from build123d import *

# Parameters (mm, degrees)
SKETCH1_W                = 3
SKETCH1_H                = 10
BOSS_EXTRUDE1_DEPTH      = 4
SKETCH2_W                = 3
SKETCH2_H                = 10
BOSS_EXTRUDE2_DEPTH      = 10
FILLET1_R                = 5
M3_CLEARANCE_HOLE1_D     = 3.4
M3_CLEARANCE_HOLE1_DEPTH = 70
M3_CLEARANCE_HOLE1_TIP   = 1.021463052
SKETCH6_W                = 10
SKETCH6_H                = 4
BOSS_EXTRUDE3_DEPTH      = 2
M3_CLEARANCE_HOLE2_D     = 3.4
M3_CLEARANCE_HOLE2_DEPTH = 70
M3_CLEARANCE_HOLE2_TIP   = 1.021463052
M3_CLEARANCE_HOLE3_D     = 3.4
M3_CLEARANCE_HOLE3_DEPTH = 70
M3_CLEARANCE_HOLE3_TIP   = 1.021463052


with BuildPart() as part:
    # Sketch1 → Boss-Extrude1 (new body)
    with BuildSketch(Plane.XY):
        Polygon((0, 15), (0, 0), (3.241791175, 0), (3.241791175, 10), (6.241791175, 10), (6.241791175, 0), (10, 0), (10, 15), align=None)
        with Locations((4.741791175, 5)):
            Rectangle(SKETCH1_W, SKETCH1_H)
    extrude(amount=BOSS_EXTRUDE1_DEPTH)

    # Sketch2 → Boss-Extrude2 (add)
    with BuildSketch(Plane.XY.offset(4)):
        with Locations((5, 5)):
            Rectangle(SKETCH2_W, SKETCH2_H)
    extrude(amount=BOSS_EXTRUDE2_DEPTH)

    # Fillet1
    fillet1_edges = [part.edges().sort_by_distance(p)[0] for p in [
        (5, 0, 14),
        (5, 10, 14),
    ]]
    fillet(fillet1_edges, radius=FILLET1_R - 0.0001)  # a hair under: the kernel refuses the full size

    # M3 Clearance Hole1
    with Locations(Plane.XY.offset(4)):
        with Locations((5, 13.5), (12.547675822, 14.055863144)):
            Hole(M3_CLEARANCE_HOLE1_D / 2, depth=M3_CLEARANCE_HOLE1_DEPTH)
            with Locations((0, 0, -(M3_CLEARANCE_HOLE1_DEPTH + M3_CLEARANCE_HOLE1_TIP / 2))):  # 118° drill point
                Cone(0, M3_CLEARANCE_HOLE1_D / 2, M3_CLEARANCE_HOLE1_TIP, mode=Mode.SUBTRACT)

    # Sketch6 → Boss-Extrude3 (add)
    with BuildSketch(Plane(origin=(0, 15, 0), x_dir=(1, 0, 0), z_dir=(0, 1, 0))):
        with Locations((5, -2)):
            Rectangle(SKETCH6_W, SKETCH6_H)
    extrude(amount=BOSS_EXTRUDE3_DEPTH)

    # M3 Clearance Hole2
    with Locations(Plane.XY.offset(4)):
        with Locations((5, 13.5)):
            Hole(M3_CLEARANCE_HOLE2_D / 2, depth=M3_CLEARANCE_HOLE2_DEPTH)
            with Locations((0, 0, -(M3_CLEARANCE_HOLE2_DEPTH + M3_CLEARANCE_HOLE2_TIP / 2))):  # 118° drill point
                Cone(0, M3_CLEARANCE_HOLE2_D / 2, M3_CLEARANCE_HOLE2_TIP, mode=Mode.SUBTRACT)

    # M3 Clearance Hole3
    with Locations(Plane(origin=(6.5, 0, 0), x_dir=(0, 0, -1), z_dir=(1, 0, 0))):
        with Locations((-10, 5)):
            Hole(M3_CLEARANCE_HOLE3_D / 2, depth=M3_CLEARANCE_HOLE3_DEPTH)
            with Locations((0, 0, -(M3_CLEARANCE_HOLE3_DEPTH + M3_CLEARANCE_HOLE3_TIP / 2))):  # 118° drill point
                Cone(0, M3_CLEARANCE_HOLE3_D / 2, M3_CLEARANCE_HOLE3_TIP, mode=Mode.SUBTRACT)


solid = part.part
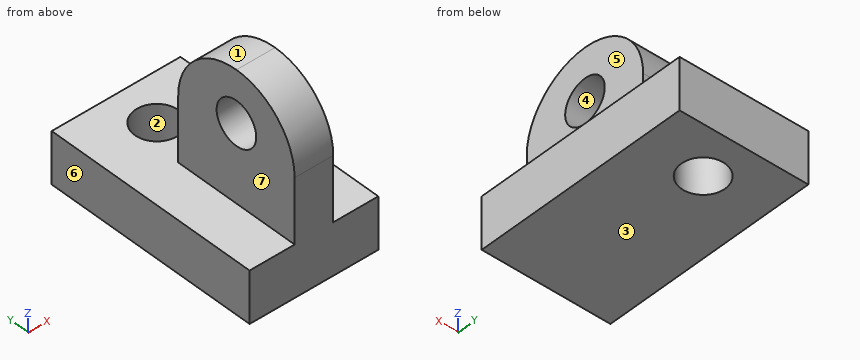
Here's how the part is built. I have some questions about the finished solid (model axes, mm). Face numbers are marked on the shaded views. A direction names the side the tool comes from. Round coordinates to 2 decimals unless told otherwise and drop trailing zeros. Write each loop counter-clockwise with the first axis right and the second up, starting at its lowest first coordinate (ties: lowest second). Pieces come first, ordered by that corner, then holes.
1. Will these pins go through, and if not, where does the flat tip stop? pin 1 Ø1.5 at (x, y) = (2, 14) entering from +Z; pin 2 Ø2.5 at (x, z) = (4.5, 6) entering from +Y; pin 3 Ø5.5 at (y, z) = (5, 10) entering from -X.
2. If we mould it in two halves opening along Z, with no side actions, what happens to the marked faces 1, 2, 3 and 4? For each: released by +Z, released by -Z, zero draft, split by the parting line, or undercut.
3. Suppose I cut it at A-A (x = 5). State how many separate pieces and enclosed holes the cut face has, and give its area (3 significant figures).
4. I need wall thicknesses on L1, parallel to Y at x = 5, z = 2.95; L2, parallel to Z at x = 7.75, y = 14.25; L3, parallel to Y at x = 6, z = 5.5. Which ranges of each line are inside material? Lowest first, please.
5. Suppose I cut it at C-C (z = 11.5). List the corners of the cut face in (x, y) for me.
6. Suppose I cut it at B-B (y = 13.5). List the corners of the cut face in (x, z) for me, and give its area (3 significant figures).
7. Suppose I cut it at D-D (z = 3.75). List the corners of the cut face in (x, y) for me, and give its area (3 significant figures).
8. For the marked faces 5, 6 and 7, which set-ups out of +Z, -Z, +X, -X, +Y, -Y let a thin tool reach every point of the face, with its end or its side?
Answer sheet:
1. pin 1: stops at z = 4
1. pin 2: stops at y = 10
1. pin 3: stops at x = 3.5
2. face 1: released by +Z
2. face 2: zero draft
2. face 3: released by -Z
2. face 4: undercut
3. separate pieces: 2
3. enclosed holes: 1
3. area: 135 mm2
4. L1: y = 0 to 11.8, 15.2 to 17
4. L2: z = 0 to 4
4. L3: y = 0 to 10
5. outline: (3.5, 0.67) - (6.5, 0.67) - (6.5, 4.2) - (3.5, 4.2) - close; (3.5, 5.8) - (6.5, 5.8) - (6.5, 9.33) - (3.5, 9.33) - close
6. outline: (0, 0) - (3.3, 0) - (3.3, 4) - (0, 4) - close; (6.7, 0) - (10, 0) - (10, 4) - (6.7, 4) - close
6. area: 26.4 mm2
7. outline: (0, 0) - (10, 0) - (10, 17) - (0, 17) - close; hole circle Ø3.4 at (5, 13.5)
7. area: 161 mm2
8. face 5: +Z, +X, +Y, -Y
8. face 6: +Z, -Z, -X, +Y, -Y
8. face 7: +Z, -X, +Y, -Y
